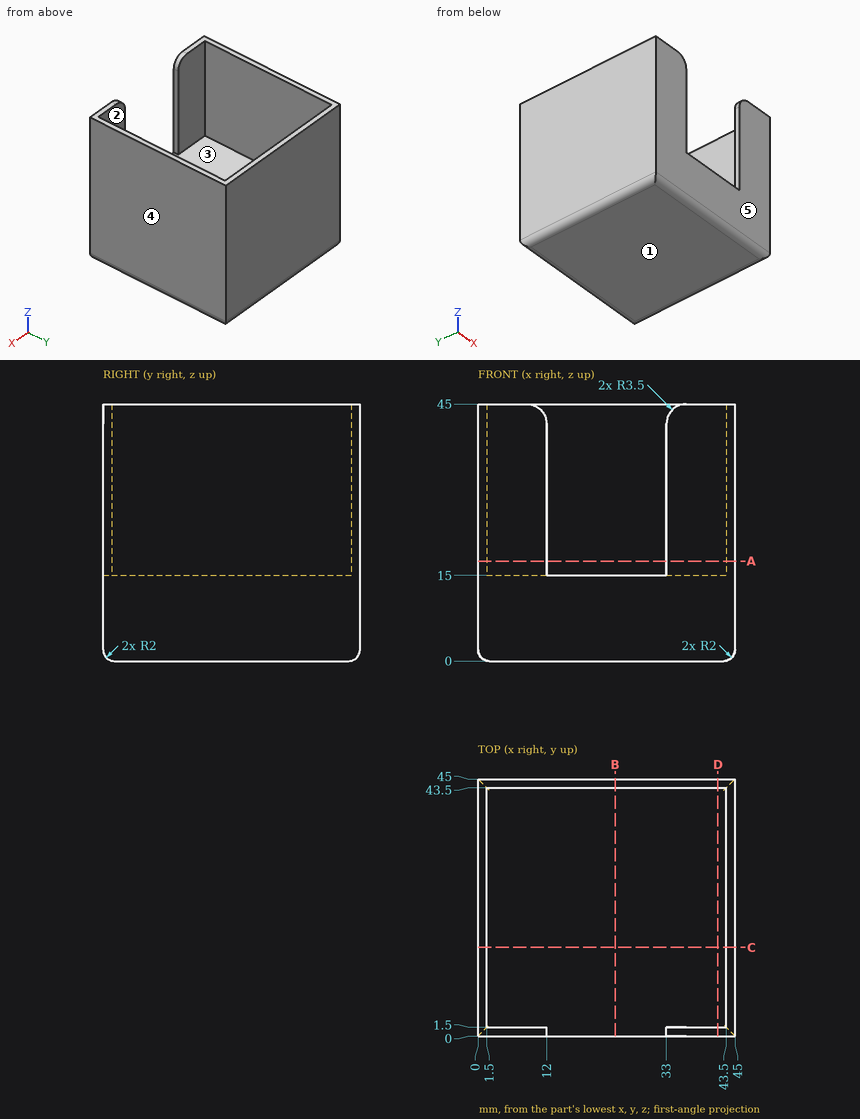
Input: dimensioned drawing with shaded views. Units: mm. Origin: part minimum x, y, z. A direction names the side the tool comes from. Round coordinates to 2 decimals unless told otherwise and drop trailing zeros. Order: outer loops, then holes, each group sorted by start corner. A loop starts at its lowest first (then second) coordinate and runs counter-clockwise, first axis right, second up. Notation, with made-up numbers: (-3, 86) -> (24, 86) arc R12 cw to (24, 96) -> close; hole circle Ø1 at (27, 25.25). An arc over 180 degrees is marked (long way). Put each result on its own line as item: value. Start each with the question number.
Q1. Line query: probe 1 along X at (y, z) = (41.5, 26); probe 2 along Y at (x, z) = (15, 17). Output: solid intervals per line, ascending.
Q2. Pull-direction query (X, two-part tool) for the marked faces 3, 4 and 5; classes: +X half, -X half, draft (parallel to the pull), parting line (faces both ways), or undercut.
Q3. Section C-C on y = 15.5. Return the cut outline in (x, z).
Q4. First-contact query: pin 1 (5 mm diameter, centred on x = 16, y = 36, fed in from +Z). Flat tip, straight axial feed; report the tip coordinate or a pass-through.
Q5. Section A-A on z = 17.5. Return the cut outline in (x, y), and give its area (4 significant figures).
Q6. Reachability of the marked faces 1 and 2 from +Z, -Z, +X, -X, +Y, -Y: full face, straight path, thin tool, end or side. Return the list, or none.
Q7. Section B-B on x = 24. Return the cut outline in (y, z).
Ans:
1. probe 1: x = 0 to 1.5, 43.5 to 45
1. probe 2: y = 43.5 to 45
2. face 3: undercut
2. face 4: +X half
2. face 5: draft
3. outline: (0, 2) arc R2 ccw to (2, 0) -> (43, 0) arc R2 ccw to (45, 2) -> (45, 45) -> (43.5, 45) -> (43.5, 15) -> (1.5, 15) -> (1.5, 45) -> (0, 45) -> close
4. pin 1: stops at z = 15
5. outline: (0, 0) -> (12, 0) -> (12, 1.5) -> (1.5, 1.5) -> (1.5, 43.5) -> (43.5, 43.5) -> (43.5, 1.5) -> (33, 1.5) -> (33, 0) -> (45, 0) -> (45, 45) -> (0, 45) -> close
5. area: 229.5 mm2
6. face 1: -Z, +X, -X, +Y, -Y
6. face 2: +Z
7. outline: (0, 2) arc R2 ccw to (2, 0) -> (43, 0) arc R2 ccw to (45, 2) -> (45, 45) -> (43.5, 45) -> (43.5, 15) -> (0, 15) -> close
